```python
from build123d import *

# Parameters (mm, degrees)
F0_R     = 7.75
F1_DEPTH = 2
F3_DEPTH = 12
F4_R     = 8
F5_DEPTH = 3
F6_R     = 0.5
F7_R     = 2.65
F8_DEPTH = 95


with BuildPart() as f1:
    # F0 (on Top) → F1 (new body)
    with BuildSketch(Plane.XY):
        Circle(F0_R)
    extrude(amount=F1_DEPTH)

    # F2 (on face) → F3 (join)
    with BuildSketch(Plane.XY.offset(2)):
        Polygon((0.5, 0), (0.5, 0.5), (0, 0.5), (-0.5, 0.5), (-0.5, 0), (-0.5, -0.5), (0, -0.5), (0.5, -0.5), align=None)
        with BuildLine():
            Line((-0.5, 0), (-0.5, 0.5))
            Line((-0.5, 0.5), (-7.7338541491, 0.5))
            ThreePointArc((-7.7338541491, 0.5), (-7.7459624856, 0.2501303103), (-7.75, 0))
            ThreePointArc((-7.75, 0), (-7.7459624856, -0.2501303103), (-7.7338541491, -0.5))
            Line((-7.7338541491, -0.5), (-0.5, -0.5))
            Line((-0.5, -0.5), (-0.5, 0))
        make_face()
        with BuildLine():
            ThreePointArc((0.5, 7.7338541491), (0.2501303103, 7.7459624856), (0, 7.75))
            ThreePointArc((0, 7.75), (-0.2501303103, 7.7459624856), (-0.5, 7.7338541491))
            Line((-0.5, 7.7338541491), (-0.5, 0.5))
            Line((-0.5, 0.5), (0, 0.5))
            Line((0, 0.5), (0.5, 0.5))
            Line((0.5, 0.5), (0.5, 7.7338541491))
        make_face()
        with BuildLine():
            Line((7.7338541491, 0.5), (0.5, 0.5))
            Line((0.5, 0.5), (0.5, 0))
            Line((0.5, 0), (0.5, -0.5))
            Line((0.5, -0.5), (7.7338541491, -0.5))
            ThreePointArc((7.7338541491, -0.5), (7.7459624856, -0.2501303103), (7.75, 0))
            ThreePointArc((7.75, 0), (7.7459624856, 0.2501303103), (7.7338541491, 0.5))
        make_face()
        with BuildLine():
            Line((0.5, -7.7338541491), (0.5, -0.5))
            Line((0.5, -0.5), (0, -0.5))
            Line((0, -0.5), (-0.5, -0.5))
            Line((-0.5, -0.5), (-0.5, -7.7338541491))
            ThreePointArc((-0.5, -7.7338541491), (-0.2501303103, -7.7459624856), (0, -7.75))
            ThreePointArc((0, -7.75), (0.2501303103, -7.7459624856), (0.5, -7.7338541491))
        make_face()
    extrude(amount=F3_DEPTH)

    # F4 (on face) → F5 (join)
    with BuildSketch(Plane.XY.offset(14)):
        Circle(F4_R)
        with BuildLine():
            Line((-7.7338541491, 0.5), (-0.5, 0.5))
            Line((-0.5, 0.5), (-0.5, 7.7338541491))
            ThreePointArc((-0.5, 7.7338541491), (0, 7.75), (0.5, 7.7338541491))
            Line((0.5, 7.7338541491), (0.5, 0.5))
            Line((0.5, 0.5), (7.7338541491, 0.5))
            ThreePointArc((7.7338541491, 0.5), (7.75, 0), (7.7338541491, -0.5))
            Line((7.7338541491, -0.5), (0.5, -0.5))
            Line((0.5, -0.5), (0.5, -7.7338541491))
            ThreePointArc((0.5, -7.7338541491), (0, -7.75), (-0.5, -7.7338541491))
            Line((-0.5, -7.7338541491), (-0.5, -0.5))
            Line((-0.5, -0.5), (-7.7338541491, -0.5))
            ThreePointArc((-7.7338541491, -0.5), (-7.75, 0), (-7.7338541491, 0.5))
        make_face(mode=Mode.SUBTRACT)
        with BuildLine():
            Line((-0.5, 7.7338541491), (-0.5, 0.5))
            Line((-0.5, 0.5), (-7.7338541491, 0.5))
            ThreePointArc((-7.7338541491, 0.5), (-7.75, 0), (-7.7338541491, -0.5))
            Line((-7.7338541491, -0.5), (-0.5, -0.5))
            Line((-0.5, -0.5), (-0.5, -7.7338541491))
            ThreePointArc((-0.5, -7.7338541491), (0, -7.75), (0.5, -7.7338541491))
            Line((0.5, -7.7338541491), (0.5, -0.5))
            Line((0.5, -0.5), (7.7338541491, -0.5))
            ThreePointArc((7.7338541491, -0.5), (7.75, 0), (7.7338541491, 0.5))
            Line((7.7338541491, 0.5), (0.5, 0.5))
            Line((0.5, 0.5), (0.5, 7.7338541491))
            ThreePointArc((0.5, 7.7338541491), (0, 7.75), (-0.5, 7.7338541491))
        make_face()
    extrude(amount=F5_DEPTH)

    # F6
    f6_edges = [f1.edges().sort_by_distance(p)[0] for p in [
        (-7.75, 0, 0),
    ]]
    fillet(f6_edges, radius=F6_R)

    # F7 (on face) → F8 (join)
    with BuildSketch(Plane.XY.offset(17)):
        Circle(F7_R)
    extrude(amount=F8_DEPTH)


solid = f1.part
```
For this review, take the finished solid that the model builds, in its own axes (mm). A direction names the side the tool comes from. Give positions to 0.01 mm unless a question says otherwise; leave off trailing zeros. Write each loop counter-clockwise with the first axis right and the second up, starting at its lowest first coordinate (ties: lowest second). Pieces come first, ordered by that corner, then holes. Notation, with made-up numbers: M -33,39.25 L -24,39.25 A13 cw -24,61.25 Z; hole C 38.25,85 d11. An arc over 180 degrees is marked long. Answer as a JSON object with one key per item and string values. Group by question number.
Item 1: For probe 1 along Z at (x, y) = (-2.25, -3); probe 2 along Z at (x, y) = (1, 1.5); probe 3 along X at (y, z) = (-0.25, 39), list the stretches that pass through material, from the lowest coordinate up. Write a range as [from, to].
Item 2: Draft analysis for pull direction Z (two halves, no side actions). For faces 6 (the flat face through (-0.5, 4, 8)), 7 (the cylindrical face through (-1.73, -7.81, 15.48)), 8 (the flat face through (0, 0, 112)), 9 (the flat face through (-3, 3, 2)), state which applies: +Z half, -Z half, draft (parallel to the pull), parting line (faces both ways), or undercut.
Item 3: Tool access review of faces 1 (the flat face through (-4, -0.5, 8)), 2 (the flat face through (2, -2, 14)), 3 (the flat face through (3, -3, 2)), 4 (the flat face through (-2, 2, 17)), 5 (the flat face through (-4, 0.5, 8)): name each direction out of +Z, -Z, +X, -X, +Y, -Y from which nothing blocks a thin tool from reaching the whole face with its end or side.
Item 4: Consider section A-A on z = 82. Write out the cut boundary in (x, y).
Item 5: For pin 1 Ø6 at (y, z) = (-3, 64.5) entering from -X; pin 2 Ø8 at (y, z) = (-0.5, 67) entering from +X; pin 3 Ø6 at (x, z) = (4, 6) entering from +Y; pin 4 Ø1 at (y, z) = (-3.5, 97) entering from -X, all flat-tipped, find the tip position at first contact; note any pin that passes through.
Check result:
{
 "1": {"probe 1": "z = [0, 2], [14, 17]", "probe 2": "z = [0, 2], [14, 112]", "probe 3": "x = [-2.64, 2.64]"},
 "2": {"face 6": "undercut", "face 7": "draft", "face 8": "+Z half", "face 9": "undercut"},
 "3": {"face 1": "-X, -Y", "face 2": "none", "face 3": "+X, -Y", "face 4": "+Z", "face 5": "-X, +Y"},
 "4": {"outline": "C 0,0 d5.3"},
 "5": {"pin 1": "stops at x = -2.65", "pin 2": "stops at x = 2.65", "pin 3": "stops at y = 0.5", "pin 4": "passes through"}
}
